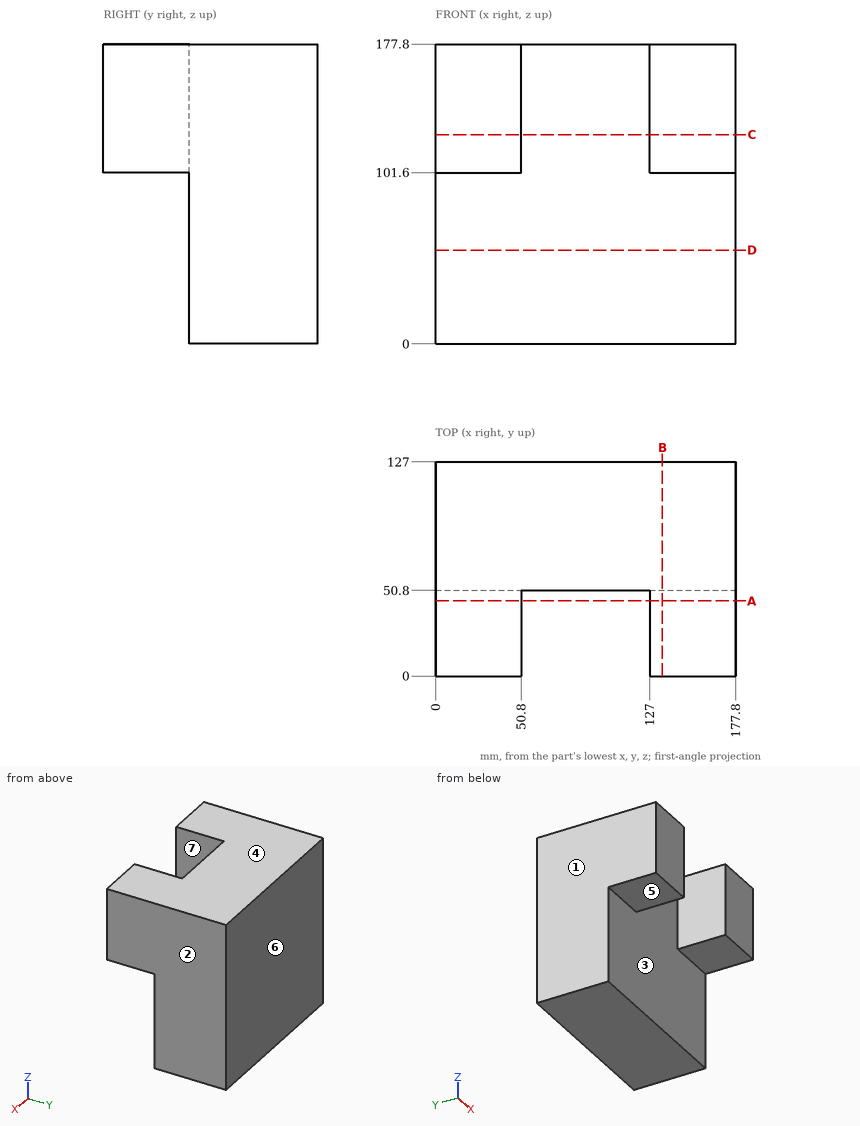
The figure shows three views and two pictorial views of one solid part (mm, origin at its lowest corner). Answer the questions. A direction names the side the tool comes from. Give positions to 0.01 mm unless a question says otherwise; leave off trailing zeros. Order: outer loops, then holes, each group sorted by start corner. A loop starts at its lowest first (then second) coordinate and runs counter-clockwise, first axis right, second up. Notation, with made-up numbers: (7.5, 65.5) -> (42.5, 65.5) arc R14 cw to (42.5, 91.5) -> close; hole circle Ø1 at (86, -33). An arc over 180 degrees is marked (long way). One line per item, written item: value.
1) Find section D-D, the plane z = 55.5. Determine the outline of the cut face in (x, y), plus the area to 3 significant figures.
Reported:
outline: (0, 50.8) -> (177.8, 50.8) -> (177.8, 127) -> (0, 127) -> close
area: 13,500 mm^2
2) Find section A-A, the plane y = 44.5. Determine the outline of the cut face in (x, z), plus the area to 3 significant figures.
Reported:
outline: (0, 101.6) -> (50.8, 101.6) -> (50.8, 177.8) -> (0, 177.8) -> close; (127, 101.6) -> (177.8, 101.6) -> (177.8, 177.8) -> (127, 177.8) -> close
area: 7,740 mm^2
3) Find section B-B, the plane x = 134.5. Determine the outline of the cut face in (y, z).
Reported:
outline: (0, 101.6) -> (50.8, 101.6) -> (50.8, 0) -> (127, 0) -> (127, 177.8) -> (0, 177.8) -> close
4) Find the intervals of material crossed by line 1 (X direction, y = 37.5, z = 142); line 2 (Z direction, x = 18, y = 43); line 3 (Y direction, x = 76, z = 101.5), in increasing order.
Reported:
line 1: x = 0 to 50.8, 127 to 177.8
line 2: z = 101.6 to 177.8
line 3: y = 50.8 to 127
5) A tool of negligible diameter and unlimited length cuts with its end or side. For the marked faces 5, 6 and 7, from which of +Z, -Z, +X, -X, +Y, -Y can it reach the whole face along a straight path? Write none if from no direction.
Reported:
face 5: -Z, +X, -X, -Y
face 6: +Z, -Z, +X, -X, +Y
face 7: +Z, -Z, -Y
6) Find section C-C, the plane z = 124. Determine the outline of the cut face in (x, y).
Reported:
outline: (0, 0) -> (50.8, 0) -> (50.8, 50.8) -> (127, 50.8) -> (127, 0) -> (177.8, 0) -> (177.8, 127) -> (0, 127) -> close
7) Determine the mould class of the marked faces 1, 2, 3 and 4 for opening direction X: pulls with the +X half, pulls with the -X half, needs draft (parallel to the pull), parting line crosses it, or undercut.
Reported:
face 1: pulls with the -X half
face 2: pulls with the +X half
face 3: undercut
face 4: needs draft
8) Flat-ended cylindrical pins translate along their axes: P1, Ø4, axis at x = 82.5, z = 123.5, coming from the -Y side; P2, Ø4, axis at x = 64.5, y = 65, coming from the -Z side. Find the tip coordinate at first contact, or state that the pin passes through.
Reported:
P1: stops at y = 50.8
P2: stops at z = 0
